Geometry check sheet. Reference: the model listing, model coordinates, mm. A direction names the side the tool comes from. Coordinates: 2 decimals unless noted, no trailing zeros. Write each loop counter-clockwise with the first axis right and the second up, starting at its lowest first coordinate (ties: lowest second). Pieces come first, ordered by that corner, then holes. Notation, with made-up numbers: (80, -27) -> (90, -27) arc R29 ccw to (90, -2) -> close; hole circle Ø1 at (-34.5, 40). An arc over 180 degrees is marked (long way). Use a Markdown table: item, result.
```python
from build123d import *

# Parameters (mm, degrees)
SKETCH1_W           = 75.411469328
SKETCH1_H           = 25.4
BOSS_EXTRUDE1_DEPTH = 12.7
SKETCH3_W           = 12.7
SKETCH3_H           = 25.4
BOSS_EXTRUDE2_DEPTH = 25.4
SKETCH4_W           = 7.642985312
SKETCH4_H           = 25.4
BOSS_EXTRUDE4_DEPTH = 25.4
SKETCH5_W           = 72.340144766
SKETCH5_H           = 25.4
CUT_EXTRUDE1_DEPTH  = 6.604
SKETCH6_W           = 20.82833925
SKETCH6_H           = 25.4
BOSS_EXTRUDE5_DEPTH = 25.4
SKETCH7_W           = 72.340144766
SKETCH7_H           = 25.4
BOSS_EXTRUDE6_DEPTH = 10.16
SKETCH8_W           = 38.1
SKETCH8_H           = 25.4
CUT_EXTRUDE2_DEPTH  = 1


with BuildPart() as part:
    # Sketch1 → Boss-Extrude1 (new body)
    with BuildSketch(Plane(origin=(0, 0, 0), x_dir=(0, 0, -1), z_dir=(1, 0, 0))):
        with Locations((37.705734664, -12.7)):
            Rectangle(SKETCH1_W, SKETCH1_H)
        Polygon((19.685, -12.7), (16.0655, -6.430842102), (8.8265, -6.430842102), (5.207, -12.7), (8.8265, -18.969157898), (16.0655, -18.969157898), align=None, mode=Mode.SUBTRACT)
    extrude(amount=BOSS_EXTRUDE1_DEPTH)

    # Sketch3 → Boss-Extrude2 (add)
    with BuildSketch(Plane(origin=(0, 0, -75.411469328), x_dir=(-1, 0, 0), z_dir=(0, 0, -1))):
        with Locations((-6.35, -12.7)):
            Rectangle(SKETCH3_W, SKETCH3_H)
    extrude(amount=BOSS_EXTRUDE2_DEPTH)

    # Sketch4 → Boss-Extrude4 (add)
    with BuildSketch(Plane.ZY):
        with Locations((-24.649831906, -12.7)):
            Rectangle(SKETCH4_W, SKETCH4_H)
    extrude(amount=BOSS_EXTRUDE4_DEPTH)

    # Sketch5 → Cut-Extrude1 (cut)
    with BuildSketch(Plane.ZY):
        with Locations((-64.641396945, -12.7)):
            Rectangle(SKETCH5_W, SKETCH5_H)
    extrude(amount=-CUT_EXTRUDE1_DEPTH, mode=Mode.SUBTRACT)

    # Sketch6 → Boss-Extrude5 (add)
    with BuildSketch(Plane.ZY):
        with Locations((-10.414169625, -12.7)):
            Rectangle(SKETCH6_W, SKETCH6_H)
        Polygon((-8.8265, -6.430842102), (-16.0655, -6.430842102), (-19.685, -12.7), (-16.0655, -18.969157898), (-8.8265, -18.969157898), (-5.207, -12.7), align=None, mode=Mode.SUBTRACT)
    extrude(amount=BOSS_EXTRUDE5_DEPTH)

    # Sketch7 → Boss-Extrude6 (add)
    with BuildSketch(Plane.ZY.offset(-6.604)):
        with Locations((-64.641396945, -12.7)):
            Rectangle(SKETCH7_W, SKETCH7_H)
    extrude(amount=BOSS_EXTRUDE6_DEPTH)

    # Sketch8 → Cut-Extrude2 (cut)
    with BuildSketch(Plane.XY):
        with Locations((-6.35, -12.7)):
            Rectangle(SKETCH8_W, SKETCH8_H)
    extrude(amount=-CUT_EXTRUDE2_DEPTH, mode=Mode.SUBTRACT)


solid = part.part
```
Item 1: Section check A-A on x = -19.5. Record the boundary of the cut face in (y, z) (1 decimal).
Answer block:
| item | result |
|---|---|
| outline | (-25.4, -28.5) -> (0, -28.5) -> (0, -1) -> (-25.4, -1) -> close; hole (-19, -16.1) -> (-12.7, -19.7) -> (-6.4, -16.1) -> (-6.4, -8.8) -> (-12.7, -5.2) -> (-19, -8.8) -> close |
Item 2: Section check C-C on z = -18. Record the boundary of the cut face in (x, y).
Answer block:
| item | result |
|---|---|
| outline | (-25.4, -25.4) -> (12.7, -25.4) -> (12.7, -15.62) -> (-25.4, -15.62) -> close; (-25.4, -9.78) -> (12.7, -9.78) -> (12.7, 0) -> (-25.4, 0) -> close |
Item 3: Tool access check on faces 5 (the flat face through (-7, -13, -1)), 6 (the flat face through (-6, -6.431, -12)), 7 (the flat face through (-3.556, -13, -65)). Record the directions out of +Z, -Z, +X, -X, +Y, -Y that give a thin tool (end or side, any length) a straight path to the whole face; none if there is none.
Answer block:
| item | result |
|---|---|
| face 5 | +Z, +X, -X, +Y, -Y |
| face 6 | +X, -X |
| face 7 | -Z, -X, +Y, -Y |
Item 4: Section check B-B on y = -10.75. Record the boundary of the cut face in (x, z), then the cut area to 3 significant figures.
Answer block:
| item | result |
|---|---|
| outline | (-25.4, -28.47) -> (-3.56, -28.47) -> (-3.56, -100.81) -> (12.7, -100.81) -> (12.7, -18.56) -> (-25.4, -18.56) -> close; (-25.4, -6.33) -> (12.7, -6.33) -> (12.7, -1) -> (-25.4, -1) -> close |
| area | 1,760 mm^2 |
Item 5: Mould release check, pull along Y, two halves, no side actions. Record for faces 1 (the flat face through (2, 0, -41)), 2 (the flat face through (-6.08, -9.52, -17.85)), 3 (the flat face through (2, -25.4, -41)), 4 (the flat face through (-25.4, -13, -21)): +Y half, -Y half, draft (parallel to the pull), parting line (faces both ways), or undercut.
Answer block:
| item | result |
|---|---|
| face 1 | +Y half |
| face 2 | undercut |
| face 3 | -Y half |
| face 4 | draft |
Item 6: Depth check by flat-ended pin: P1, Ø7.5, axis at y = -7, z = -67.5, coming from the -X side; P2, Ø3.5, axis at x = 0, z = -12.5, coming from the +Y side; P3, Ø3, axis at x = -17.5, y = -8.5, coming from the -Z side; P4, Ø1, axis at x = -4.5, z = -53.5, coming from the +Y side. Enter the tip coordinate at first touch or a pass-through.
Answer block:
| item | result |
|---|---|
| P1 | stops at x = -3.56 |
| P2 | stops at y = 0 |
| P3 | stops at z = -28.47 |
| P4 | passes through |
Item 7: Section check D-D on y = -5.25. Record the boundary of the cut face in (x, z).
Answer block:
| item | result |
|---|---|
| outline | (-25.4, -28.47) -> (-3.56, -28.47) -> (-3.56, -100.81) -> (12.7, -100.81) -> (12.7, -1) -> (-25.4, -1) -> close |
Item 8: Thickness scan on L1, parallel to X at y = -23.75, z = -30; L2, parallel to Z at x = -21, y = -3; L3, parallel to Z at x = -18, y = -14. Record the ranges inside material, lowest first. Write a range as [from, to].
Answer block:
| item | result |
|---|---|
| L1 | x = [-3.56, 12.7] |
| L2 | z = [-28.47, -1] |
| L3 | z = [-28.47, -18.93], [-5.96, -1] |
